For this review, take the finished solid that the model builds, in its own axes (mm). Give positions to 0.01 mm unless a question says otherwise; leave off trailing zeros. Loops run counter-clockwise (first coordinate to the right, second up) from the corner with the lowest first, then second, coordinate; pieces in that order, holes last.
```python
from build123d import *

# Parameters (mm, degrees)
SKETCH1_R      = 13.6144
EXTRUDE1_DEPTH = 609.6


with BuildPart() as part:
    # Sketch1 → Extrude1 (new body)
    with BuildSketch(Plane.XY):
        with BuildLine():
            Line((-4.287037938, 26.9748), (4.287037938, 26.9748))
            Line((4.287037938, 26.9748), (23.0759, 16.127045431))
            ThreePointArc((23.0759, 16.127045431), (24.191545431, 15.0114), (24.5999, 13.4874))
            Line((24.5999, 13.4874), (24.5999, -14.538760091))
            ThreePointArc((24.5999, -14.538760091), (0, -28.575), (-24.5999, -14.538760091))
            Line((-24.5999, -14.538760091), (-24.5999, 13.4874))
            ThreePointArc((-24.5999, 13.4874), (-24.191545431, 15.0114), (-23.0759, 16.127045431))
            Line((-23.0759, 16.127045431), (-4.287037938, 26.9748))
        make_face()
        Circle(SKETCH1_R, mode=Mode.SUBTRACT)
    extrude(amount=-EXTRUDE1_DEPTH)


solid = part.part
```
Item 1: Take a section at B-B on y = 0. Give the boundary of the cut face in (x, z), and give its area (3 significant figures).
Answer:
outline: (-24.6, -609.6) - (-13.61, -609.6) - (-13.61, 0) - (-24.6, 0) - close; (13.61, -609.6) - (24.6, -609.6) - (24.6, 0) - (13.61, 0) - close
area: 13,400 mm2
Item 2: The part is to be moulded in two halves that separate along X. For faces 1 (the flat face through (-13.813, 21.475, -300.533)), 2 (the cylindrical face through (12.58, -5.21, -300.53)), 3 (the flat face through (6, -13, -609.6)), 4 (the flat face through (13.55, 21.627, -300.533)), say which applies: released by +X, released by -X, zero draft, split by the parting line, or undercut.
Answer:
face 1: released by -X
face 2: undercut
face 3: zero draft
face 4: released by +X
Item 3: For L1, parallel to Y at x = 0, z = -475 (3 decimals); L2, parallel to X at y = -1, z = -116.5; L3, parallel to Y at x = 5.5, z = -44.5, list the stretches that pass through material, from the lowest coordinate up.
Answer:
L1: y = -28.575 to -13.614, 13.614 to 26.975
L2: x = -24.6 to -13.58, 13.58 to 24.6
L3: y = -28.04 to -12.45, 12.45 to 26.27
Item 4: Clearance check with flat-ended pins moving along their axes: pin 1 Ø1.5 at (y, z) = (-23, -486.5) entering from -X; pin 2 Ø10 at (x, z) = (2.5, -100) entering from -Y (3 decimals); pin 3 Ø3 at (x, z) = (9, -181.5) entering from +Y. State where each tip first meets the part, or that it passes through.
Answer:
pin 1: stops at x = -17.93
pin 2: stops at y = -28.575
pin 3: stops at y = 25.12
Item 5: Take a section at A-A on z = -457. Give the boundary of the cut face in (x, y) (3 decimals).
Answer:
outline: (-24.6, -14.539) arc R28.575 ccw to (24.6, -14.539) - (24.6, 13.487) arc R3.048 ccw to (23.076, 16.127) - (4.287, 26.975) - (-4.287, 26.975) - (-23.076, 16.127) arc R3.048 ccw to (-24.6, 13.487) - close; hole circle Ø27.229 at (0, 0)
